from build123d import *

# Parameters (mm, degrees)
SKETCH1_W           = 130
SKETCH1_H           = 130
SKETCH1_R           = 2.5
SKETCH1_W_2         = 4
SKETCH1_H_2         = 30
BOSS_EXTRUDE1_DEPTH = 3
FILLET1_R           = 5
FILLET2_R           = 2


with BuildPart() as part:
    # Sketch1 → Boss-Extrude1 (new body)
    with BuildSketch(Plane(origin=(0, 0, 0), x_dir=(1, 0, 0), z_dir=(0, 1, 0))):
        Rectangle(SKETCH1_W, SKETCH1_H)
        with Locations(Location((-52.5, 52.5, 0), (0, 0, 270))):
            Circle(SKETCH1_R, mode=Mode.SUBTRACT)
        with Locations(Location((-34.82233047, 34.82233047, 0), (0, 0, 270))):
            Circle(SKETCH1_R, mode=Mode.SUBTRACT)
        with Locations(Location((52.5, 52.5, 0), (0, 0, 270))):
            Circle(SKETCH1_R, mode=Mode.SUBTRACT)
        with Locations(Location((34.82233047, 34.82233047, 0), (0, 0, 270))):
            Circle(SKETCH1_R, mode=Mode.SUBTRACT)
        with Locations(Location((52.5, -52.5, 0), (0, 0, 90))):
            Circle(SKETCH1_R, mode=Mode.SUBTRACT)
        with Locations(Location((34.82233047, -34.82233047, 0), (0, 0, 90))):
            Circle(SKETCH1_R, mode=Mode.SUBTRACT)
        with Locations(Location((-34.82233047, -34.82233047, 0), (0, 0, 90))):
            Circle(SKETCH1_R, mode=Mode.SUBTRACT)
        with Locations(Location((-52.5, -52.5, 0), (0, 0, 90))):
            Circle(SKETCH1_R, mode=Mode.SUBTRACT)
        with Locations((-23, 25)):
            Rectangle(SKETCH1_W_2, SKETCH1_H_2, mode=Mode.SUBTRACT)
        with Locations((23, 25)):
            Rectangle(SKETCH1_W_2, SKETCH1_H_2, mode=Mode.SUBTRACT)
        with Locations((23, -25)):
            Rectangle(SKETCH1_W_2, SKETCH1_H_2, mode=Mode.SUBTRACT)
        with Locations((-23, -25)):
            Rectangle(SKETCH1_W_2, SKETCH1_H_2, mode=Mode.SUBTRACT)
    extrude(amount=BOSS_EXTRUDE1_DEPTH)

    # Fillet1
    fillet1_edges = [part.edges().sort_by_distance(p)[0] for p in [
        (65, 1.5, 65),
        (-65, 1.5, 65),
        (-65, 1.5, -65),
        (65, 1.5, -65),
    ]]
    fillet(fillet1_edges, radius=FILLET1_R)

    # Fillet2
    fillet2_edges = [part.edges().sort_by_distance(p)[0] for p in [
        (-25, 1.5, 40),
        (-21, 1.5, 40),
        (-25, 1.5, 10),
        (-21, 1.5, 10),
        (-21, 1.5, -10),
        (-25, 1.5, -10),
        (-25, 1.5, -40),
        (-21, 1.5, -40),
        (25, 1.5, -40),
        (21, 1.5, -40),
        (21, 1.5, -10),
        (25, 1.5, -10),
        (21, 1.5, 10),
        (25, 1.5, 10),
        (21, 1.5, 40),
        (25, 1.5, 40),
    ]]
    fillet(fillet2_edges, radius=FILLET2_R - 0.0001)  # a hair under: the kernel refuses the full size


solid = part.part
Input: part model. Units: mm. Frame: model coordinates. A direction names the side the tool comes from. Round coordinates to 2 decimals unless told otherwise and drop trailing zeros. Order: outer loops, then holes, each group sorted by start corner. A loop starts at its lowest first (then second) coordinate and runs counter-clockwise, first axis right, second up.
1. Material intervals for line 1 (X direction, y = 2.1, z = -35); line 2 (X direction, y = 2.4, z = 52.5); line 3 (X direction, y = 1.8, z = 23.5), sorted ascending.
The answers:
line 1: x = -65 to -37.32, -32.33 to -25, -21 to 21, 25 to 32.33, 37.32 to 65
line 2: x = -65 to -55, -50 to 50, 55 to 65
line 3: x = -65 to -25, -21 to 21, 25 to 65
2. Mould query, pull axis X, two halves, no side actions, for faces 1 (the face through (21, 1, -25)), 2 (the face through (-1, 1, 65)), 3 (the face through (-65, 1, 1)), 4 (the face through (63, 2, -64)). Classes: released by +X, released by -X, zero draft, split by the parting line, or undercut.
The answers:
face 1: undercut
face 2: zero draft
face 3: released by -X
face 4: released by +X
3. Cut plane A-A, the plane x = 52.5. Output: boundary loops of the cut face in (y, z), then the cut area to 3 significant figures.
The answers:
outline: (0, -65) - (3, -65) - (3, -55) - (0, -55) - close; (0, -50) - (3, -50) - (3, 50) - (0, 50) - close; (0, 55) - (3, 55) - (3, 65) - (0, 65) - close
area: 360 mm2
4. Cut plane B-B, the plane z = 52.5. Output: boundary loops of the cut face in (x, y), then the cut area to 3 significant figures.
The answers:
outline: (-65, 0) - (-55, 0) - (-55, 3) - (-65, 3) - close; (-50, 0) - (50, 0) - (50, 3) - (-50, 3) - close; (55, 0) - (65, 0) - (65, 3) - (55, 3) - close
area: 360 mm2
5. Set-up query: faces 5 (the face through (-21, 1, 25)), 6 (the face through (63, 2, 64)). Return all of +Z, -Z, +X, -X, +Y, -Y with unobstructed straight access to the full face (end or side cutting, diameter ignored); none if empty.
The answers:
face 5: +Y, -Y
face 6: +Z, +X, +Y, -Y
6. Cut plane C-C, the plane y = 1.15. State how many separate pieces and enclosed holes the cut face has, then the cut area to 3 significant figures.
The answers:
separate pieces: 1
enclosed holes: 12
area: 16,300 mm2
7. Pin query (flat end, axial travel): P1, Ø3, axis at x = -34.82, z = -34.82, coming from the -Y side. Return the tip coordinate at first contact, or that it passes through.
The answers:
P1: passes through
